Can you work these out from the model? Positions are in its coordinate system, mm. A direction names the side the tool comes from. Give positions to 0.01 mm unless a question says otherwise; leave off trailing zeros. Write each loop counter-clockwise with the first axis right and the second up, starting at its lowest first coordinate (ties: lowest second). Pieces come first, ordered by that corner, then holes. Notation, with made-up numbers: (18.5, -22.5) - (36.5, -22.5) arc R27 ccw to (36.5, -4.5) - close; hole circle Ø10 at (-38.5, 49). An arc over 180 degrees is marked (long way). Use a Markdown table: item, result. Add a question column.
```python
from build123d import *

# Parameters (mm, degrees)
BOSS_EXTRUDE1_DEPTH = 19
SKETCH3_R           = 4.01
CUT_EXTRUDE1_DEPTH  = 29.952983186
BOSS_EXTRUDE2_START = 6
SKETCH5_R           = 9
SKETCH5_R_2         = 4.01
BOSS_EXTRUDE2_DEPTH = 6
SKETCH6_W           = 2
SKETCH6_H           = 3.816021538
CUT_EXTRUDE3_DEPTH  = 34.200530649
SKETCH10_W          = 1.25
SKETCH10_H          = 12.389397068


with BuildPart() as part:
    # Sketch2 → Boss-Extrude1 (new body)
    with BuildSketch(Plane(origin=(0, 0, 0), x_dir=(1, 0, 0), z_dir=(0, 1, 0))):
        with BuildLine():
            Line((7.335535963, -10.343914335), (9.974123377, -8.426868365))
            Line((9.974123377, -8.426868365), (11.654796972, -9.560497019))
            ThreePointArc((11.654796972, -9.560497019), (13.098043776, -7.864477351), (14.265066544, -5.967769174))
            Line((14.265066544, -5.967769174), (12.667564922, -4.719664118))
            Line((12.667564922, -4.719664118), (13.675415632, -1.617818581))
            Line((13.675415632, -1.617818581), (15.701439337, -1.547068275))
            ThreePointArc((15.701439337, -1.547068275), (15.87215518, 0.673359646), (15.701439337, 2.893787567))
            Line((15.701439337, 2.893787567), (13.675415632, 2.964537874))
            Line((13.675415632, 2.964537874), (12.667564922, 6.066383411))
            Line((12.667564922, 6.066383411), (14.265066544, 7.314488466))
            ThreePointArc((14.265066544, 7.314488466), (13.098043776, 9.211196644), (11.654796972, 10.907216312))
            Line((11.654796972, 10.907216312), (9.974123377, 9.773587658))
            Line((9.974123377, 9.773587658), (7.335535963, 11.690633627))
            Line((7.335535963, 11.690633627), (7.894324179, 13.639359722))
            ThreePointArc((7.894324179, 13.639359722), (5.835325832, 14.487870099), (3.670819293, 15.011659646))
            Line((3.670819293, 15.011659646), (2.977455996, 13.106659646))
            Line((2.977455996, 13.106659646), (-0.284017411, 13.106659646))
            Line((-0.284017411, 13.106659646), (-0.977380707, 15.011659646))
            ThreePointArc((-0.977380707, 15.011659646), (-3.141887247, 14.487870099), (-5.200885594, 13.639359722))
            Line((-5.200885594, 13.639359722), (-4.642097378, 11.690633627))
            Line((-4.642097378, 11.690633627), (-7.280684791, 9.773587658))
            Line((-7.280684791, 9.773587658), (-8.961358387, 10.907216312))
            ThreePointArc((-8.961358387, 10.907216312), (-10.40460519, 9.211196644), (-11.571627958, 7.314488466))
            Line((-11.571627958, 7.314488466), (-9.974126336, 6.066383411))
            Line((-9.974126336, 6.066383411), (-10.981977046, 2.964537874))
            Line((-10.981977046, 2.964537874), (-13.008000751, 2.893787567))
            ThreePointArc((-13.008000751, 2.893787567), (-13.178716594, 0.673359646), (-13.008000751, -1.547068275))
            Line((-13.008000751, -1.547068275), (-10.981977046, -1.617818581))
            Line((-10.981977046, -1.617818581), (-9.974126336, -4.719664118))
            Line((-9.974126336, -4.719664118), (-11.571627958, -5.967769174))
            ThreePointArc((-11.571627958, -5.967769174), (-10.40460519, -7.864477351), (-8.961358387, -9.560497019))
            Line((-8.961358387, -9.560497019), (-7.280684791, -8.426868365))
            Line((-7.280684791, -8.426868365), (-4.642097378, -10.343914335))
            Line((-4.642097378, -10.343914335), (-5.200885594, -12.292640429))
            ThreePointArc((-5.200885594, -12.292640429), (-3.141887247, -13.141150806), (-0.977380707, -13.664940354))
            Line((-0.977380707, -13.664940354), (-0.284017411, -11.759940354))
            Line((-0.284017411, -11.759940354), (2.977455996, -11.759940354))
            Line((2.977455996, -11.759940354), (3.670819293, -13.664940354))
            ThreePointArc((3.670819293, -13.664940354), (5.835325832, -13.141150806), (7.894324179, -12.292640429))
            Line((7.894324179, -12.292640429), (7.335535963, -10.343914335))
        make_face()
    extrude(amount=BOSS_EXTRUDE1_DEPTH)

    # Sketch3 → Cut-Extrude1 (cut, through all)
    with BuildSketch(Plane(origin=(0, 19, 0), x_dir=(1, 0, 0), z_dir=(0, 1, 0))):
        with Locations(Location((1.346719293, 0.673359646, 0), (0, 0, 270))):
            Circle(SKETCH3_R)
    extrude(amount=-CUT_EXTRUDE1_DEPTH, mode=Mode.SUBTRACT)

    # Sketch5 → Boss-Extrude2 (add)
    with BuildSketch(Plane(origin=(0, 19, 0), x_dir=(1, 0, 0), z_dir=(0, 1, 0)).offset(BOSS_EXTRUDE2_START)):
        with Locations(Location((1.346719293, 0.673359646, 0), (0, 0, 270))):
            Circle(SKETCH5_R)
        with Locations(Location((1.346719293, 0.673359646, 0), (0, 0, 270))):
            Circle(SKETCH5_R_2, mode=Mode.SUBTRACT)
    extrude(amount=-BOSS_EXTRUDE2_DEPTH)

    # Sketch6 → Cut-Extrude3 (cut, through all)
    with BuildSketch(Plane(origin=(0, 25, 0), x_dir=(1, 0, 0), z_dir=(0, 1, 0))):
        with Locations((1.346719293, -2.367532517)):
            Rectangle(SKETCH6_W, SKETCH6_H)
    extrude(amount=-CUT_EXTRUDE3_DEPTH, mode=Mode.SUBTRACT)

    # Sketch10 → M3x0.5 Tapped Hole2 (revolve, cut)
    with BuildSketch(Plane(origin=(1.346719293, 16.7, 1.275543286), x_dir=(0, 1, 0), z_dir=(1, 0, 0))):
        with Locations((0.625, 6.194698534)):
            Rectangle(SKETCH10_W, SKETCH10_H)
    revolve(axis=Axis((1.346719293, 16.7, -5.074456714), (0, 0, 1)), mode=Mode.SUBTRACT)


solid = part.part
```
Q1. Suppose I cut it at A-A (z = -0.5). Please give me the cut outline in (x, y).
Q2. Suppose I cut it at D-D (x = 6.5). Please give me the cut outline in (y, z).
Q3. On a 3-axis mill with a long thin cutter (end or side, diameter ignored), from which of +Z, -Z, +X, -X, +Y, -Y can I reach the whole of each face in a straight line? I mean faces 5 (the flat face through (1, 9, -13.107)), 6 (the flat face through (1, 8, 4.276)), 7 (the flat face through (13.164, 9.367, 3.19)). Say none if no direction works.
Q4. I'm going to push flat-ended pins straight in: P1, Ø3, axis at x = 1.35, y = 16.7, coming from the -Z side; P2, Ø1.2, axis at y = 19.5, z = 3.5, coming from the +X side; P3, Ø6, axis at x = 8, y = 17, coming from the -Z side. Where does each tip first touch, or does it pass through?
Q5. If I drill on probe 1 along X at (y, z) = (16.7, 9); probe 2 along Z at (x, y) = (-11.25, 15.75); probe 3 along Z at (x, y) = (0.75, 4), over which ranges is the centre line in solid material (lowest first)? Write a range as [from, to].
Q6. Suppose I cut it at C-C (y = 22.25). Please give me the cut outline in (x, z).
Q7. Suppose I cut it at B-B (x = -6). Please give me the cut outline in (y, z).
Q8. If we mould it in two halves opening along X, with no side actions, what happens to faces 1 (the flat face through (8, 19, -7)), 2 (the cylindrical face through (15.872, 9.367, -0.642)), 3 (the flat face through (-10.47, 9.37, -4.54)), 4 (the cylindrical face through (1.825, 17.855, 7.509))? For each: released by +X, released by -X, zero draft, split by the parting line, or undercut.
Derived:
| question | item | result |
|---|---|---|
| 1 | outline | (-13.18, 0) - (-2.66, 0) - (-2.66, 25) - (-7.65, 25) - (-7.65, 19) - (-13.18, 19) - close; (5.35, 0) - (15.87, 0) - (15.87, 19) - (10.35, 19) - (10.35, 25) - (5.35, 25) - close |
| 2 | outline | (0, -14.25) - (19, -14.25) - (19, -8.05) - (25, -8.05) - (25, 6.71) - (19, 6.71) - (19, 12.91) - (0, 12.91) - close |
| 3 | face 5 | -Z, +Y, -Y |
| 3 | face 6 | +Y, -Y |
| 3 | face 7 | +X, +Y, -Y |
| 4 | P1 | z = -13.11 |
| 4 | P2 | x = 13.17 |
| 4 | P3 | z = -14.73 |
| 5 | probe 1 | [-9.49, -8.13], [-6.49, 0.1], [2.6, 9.19], [10.82, 12.18] |
| 5 | probe 2 | [-7.91, -7.06], [-2.96, 1.61], [5.72, 6.56] |
| 5 | probe 3 | [-13.11, -4.64], [4.28, 11.76] |
| 6 | outline | circle Ø18 at (1.35, -0.67); hole (0.35, 3.21) arc R4.01 ccw (long way) to (2.35, 3.21) - (2.35, 4.28) - (0.35, 4.28) - close |
| 7 | outline | (0, -10.7) - (19, -10.7) - (19, -5.87) - (25, -5.87) - (25, 4.53) - (19, 4.53) - (19, 9.36) - (0, 9.36) - close |
| 8 | face 1 | zero draft |
| 8 | face 2 | released by +X |
| 8 | face 3 | released by -X |
| 8 | face 4 | undercut |
